The model under review builds one solid part; all positions refer to its coordinate system, in mm. A direction names the side the tool comes from. Round coordinates to 2 decimals unless told otherwise and drop trailing zeros. Write each loop counter-clockwise with the first axis right and the second up, starting at its lowest first coordinate (ties: lowest second). Pieces come first, ordered by that corner, then holes. Notation, with made-up numbers: (-30, 18.5) - (-17, 18.5) arc R30 cw to (-17, 51.5) - close; hole circle Ø2 at (-11, 89.5). An arc over 180 degrees is marked (long way). Return JSON: item names as keys, results as strings.
from build123d import *

# Parameters (mm, degrees)
SKETCH_1_W          = 100
SKETCH_1_H          = 30
SKETCH_1_R          = 1.5
SKETCH_1_W_2        = 15
SKETCH_1_H_2        = 2
SKETCH_1_W_3        = 30
SKETCH_1_H_3        = 15
EXTRUDE_1_DEPTH     = 3.2
CUT_EXTRUDE_START   = 3.2
CUT_EXTRUDE_1_DEPTH = 1.8
CHAMFER_1_SIZE      = 4
SKETCH_2_W          = 8
SKETCH_2_H          = 0.8
CUT_EXTRUDE_2_DEPTH = 53.299521986
EXTRUDE_START       = 3
SKETCH_3_R          = 2.75
SKETCH_3_W          = 30
SKETCH_3_H          = 15
SKETCH_3_W_2        = 15
SKETCH_3_H_2        = 2
SKETCH_3_R_2        = 1.5
EXTRUDE_2_DEPTH     = 3


with BuildPart() as part:
    # 스케치1 → 보스-돌출1 (new body)
    with BuildSketch(Plane(origin=(0, 0, 0), x_dir=(1, 0, 0), z_dir=(0, 1, 0))):
        Rectangle(SKETCH_1_W, SKETCH_1_H)
        with Locations(Location((0, 9.5, 0), (0, 0, 270))):
            Circle(SKETCH_1_R, mode=Mode.SUBTRACT)
        with Locations(Location((0, -9.5, 0), (0, 0, 270))):
            Circle(SKETCH_1_R, mode=Mode.SUBTRACT)
        with Locations((-16.5, 10)):
            Rectangle(SKETCH_1_W_2, SKETCH_1_H_2, mode=Mode.SUBTRACT)
        with Locations((25, 0)):
            Rectangle(SKETCH_1_W_3, SKETCH_1_H_3, mode=Mode.SUBTRACT)
        with Locations((-36.5, 10)):
            Rectangle(SKETCH_1_W_2, SKETCH_1_H_2, mode=Mode.SUBTRACT)
        with Locations((-36.5, 5)):
            Rectangle(SKETCH_1_W_2, SKETCH_1_H_2, mode=Mode.SUBTRACT)
        with Locations((-16.5, 5)):
            Rectangle(SKETCH_1_W_2, SKETCH_1_H_2, mode=Mode.SUBTRACT)
        with Locations((-36.5, 0)):
            Rectangle(SKETCH_1_W_2, SKETCH_1_H_2, mode=Mode.SUBTRACT)
        with Locations((-16.5, 0)):
            Rectangle(SKETCH_1_W_2, SKETCH_1_H_2, mode=Mode.SUBTRACT)
        with Locations((-36.5, -5)):
            Rectangle(SKETCH_1_W_2, SKETCH_1_H_2, mode=Mode.SUBTRACT)
        with Locations((-16.5, -5)):
            Rectangle(SKETCH_1_W_2, SKETCH_1_H_2, mode=Mode.SUBTRACT)
        with Locations((-36.5, -10)):
            Rectangle(SKETCH_1_W_2, SKETCH_1_H_2, mode=Mode.SUBTRACT)
        with Locations((-16.5, -10)):
            Rectangle(SKETCH_1_W_2, SKETCH_1_H_2, mode=Mode.SUBTRACT)
    extrude(amount=EXTRUDE_1_DEPTH)

    # 스케치1<3> → 컷-돌출1 (cut)
    with BuildSketch(Plane(origin=(0, 0, 0), x_dir=(1, 0, 0), z_dir=(0, 1, 0)).offset(CUT_EXTRUDE_START)):
        Polygon((0, 6.4977786), (2.6, 7.9988893), (2.6, 11.0011107), (0, 12.5022214), (-2.6, 11.0011107), (-2.6, 7.9988893), align=None)
        Polygon((2.6, -7.9988893), (0, -6.4977786), (-2.6, -7.9988893), (-2.6, -11.0011107), (0, -12.5022214), (2.6, -11.0011107), align=None)
    extrude(amount=-CUT_EXTRUDE_1_DEPTH, mode=Mode.SUBTRACT)

    # 모따기1
    chamfer_1_edges = [part.edges().sort_by_distance(p)[0] for p in [
        (-50, 1.6, 15),
        (-50, 1.6, -15),
        (50, 1.6, -15),
        (50, 1.6, 15),
    ]]
    chamfer(chamfer_1_edges, length=CHAMFER_1_SIZE)

    # 스케치2 → 컷-돌출2 (cut, through all)
    with BuildSketch(Plane(origin=(0, 3.2, 0), x_dir=(1, 0, 0), z_dir=(0, 1, 0))):
        with Locations((0, 14.6)):
            Rectangle(SKETCH_2_W, SKETCH_2_H)
        with Locations((0, -14.6)):
            Rectangle(SKETCH_2_W, SKETCH_2_H)
    extrude(amount=-CUT_EXTRUDE_2_DEPTH, mode=Mode.SUBTRACT)

    # 스케치3 → 보스-돌출2 (add)
    # profile 1 of 3: a face of its own
    with BuildSketch(Plane.XZ.offset(EXTRUDE_START)):
        Polygon((4, 14.2), (-4, 14.2), (-4, 15), (-46, 15), (-50, 11), (-50, -11), (-46, -15), (-4, -15), (-4, -14.2), (4, -14.2), (4, -15), (46, -15), (50, -11), (50, 11), (46, 15), (4, 15), align=None)
        with Locations(Location((0, 9.5, 0), (0, 0, 270))):
            Circle(SKETCH_3_R, mode=Mode.SUBTRACT)
        with Locations(Location((0, -9.5, 0), (0, 0, 270))):
            Circle(SKETCH_3_R, mode=Mode.SUBTRACT)
        with Locations((25, 0)):
            Rectangle(SKETCH_3_W, SKETCH_3_H, mode=Mode.SUBTRACT)
        with Locations((-36.5, 10)):
            Rectangle(SKETCH_3_W_2, SKETCH_3_H_2, mode=Mode.SUBTRACT)
        with Locations((-36.5, 5)):
            Rectangle(SKETCH_3_W_2, SKETCH_3_H_2, mode=Mode.SUBTRACT)
        with Locations((-36.5, 0)):
            Rectangle(SKETCH_3_W_2, SKETCH_3_H_2, mode=Mode.SUBTRACT)
        with Locations((-36.5, -5)):
            Rectangle(SKETCH_3_W_2, SKETCH_3_H_2, mode=Mode.SUBTRACT)
        with Locations((-36.5, -10)):
            Rectangle(SKETCH_3_W_2, SKETCH_3_H_2, mode=Mode.SUBTRACT)
        with Locations((-16.5, -10)):
            Rectangle(SKETCH_3_W_2, SKETCH_3_H_2, mode=Mode.SUBTRACT)
        with Locations((-16.5, -5)):
            Rectangle(SKETCH_3_W_2, SKETCH_3_H_2, mode=Mode.SUBTRACT)
        with Locations((-16.5, 0)):
            Rectangle(SKETCH_3_W_2, SKETCH_3_H_2, mode=Mode.SUBTRACT)
        with Locations((-16.5, 5)):
            Rectangle(SKETCH_3_W_2, SKETCH_3_H_2, mode=Mode.SUBTRACT)
        with Locations((-16.5, 10)):
            Rectangle(SKETCH_3_W_2, SKETCH_3_H_2, mode=Mode.SUBTRACT)
    # profile 2 of 3: a face of its own
    with BuildSketch(Plane.XZ.offset(EXTRUDE_START)):
        with Locations(Location((0, -9.5, 0), (0, 0, 270))):
            Circle(SKETCH_3_R_2)
    # profile 3 of 3: a face of its own
    with BuildSketch(Plane.XZ.offset(EXTRUDE_START)):
        with Locations(Location((0, 9.5, 0), (0, 0, 270))):
            Circle(SKETCH_3_R_2)
    extrude(amount=-EXTRUDE_2_DEPTH)


with BuildPart() as extrude_2_kept_piece:
    # of the separate pieces the step leaves, the one the design keeps (extrude_2_pieces_kept)
    add(part.part.solids().sort_by_distance((-4, -3, 15))[0])


solid = extrude_2_kept_piece.part
(1) Add section A-A (z = -2). Write out the cut boundary in (x, y).
Filled in:
{"outline": "(-50, -3) - (10, -3) - (10, 3.2) - (-50, 3.2) - close; (40, -3) - (50, -3) - (50, 3.2) - (40, 3.2) - close"}
(2) Mouldability with a two-part tool opening along X and no side actions: class faces 1 (the flat face through (-37, 0, 9)), 2 (the flat face through (-50, 0, 0)) as released by +X, released by -X, zero draft, split by the parting line, or undercut.
Filled in:
{"face 1": "undercut", "face 2": "released by -X"}
(3) Wall thickness on line 1 (Z direction, x = 0, y = 0.6); line 2 (X direction, y = 0.5, z = 5); line 3 (Z direction, x = -20, y = -2): over which ranges is each line inside the solid? List them lowest first.
Filled in:
{"line 1": "z = -14.2 to -11, -8 to 8, 11 to 14.2", "line 2": "x = -50 to -44, -29 to -24, -9 to 10, 40 to 50", "line 3": "z = -15 to -11, -9 to -6, -4 to -1, 1 to 4, 6 to 9, 11 to 15"}
(4) Add section B-B (x = -11.5). Write out the cut boundary in (y, z).
Filled in:
{"outline": "(-3, -15) - (3.2, -15) - (3.2, -11) - (-3, -11) - close; (-3, -9) - (3.2, -9) - (3.2, -6) - (-3, -6) - close; (-3, -4) - (3.2, -4) - (3.2, -1) - (-3, -1) - close; (-3, 1) - (3.2, 1) - (3.2, 4) - (-3, 4) - close; (-3, 6) - (3.2, 6) - (3.2, 9) - (-3, 9) - close; (-3, 11) - (3.2, 11) - (3.2, 15) - (-3, 15) - close"}
(5) Clearance check with flat-ended pins moving along their axes: pin 1 Ø1.6 at (x, z) = (1, -9) entering from -Y; pin 2 Ø1 at (x, z) = (13.5, 6) entering from -Y. State where each tip first meets the part, or that it passes through.
Filled in:
{"pin 1": "stops at y = 0", "pin 2": "passes through"}
(6) For faces 3 (the flat face through (1.282, 2.313, 11.762)), 4 (the flat face through (-44, 0, -10)), 5 (the flat face through (0, 0, -14.2)), 6 (the cylindrical face through (-1.05, -1.52, 6.96)), list the 3-axis set-ups (+Z, -Z, +X, -X, +Y, -Y) from which the entire face can be reached by the end or side of a thin tool; tool diameter is ignored.
Filled in:
{"face 3": "+Y", "face 4": "+Y, -Y", "face 5": "-Z, +Y, -Y", "face 6": "-Y"}
